Autodesk Inventor part; units mm, degrees
ref_plane "YZ Plane" through (0, 0, 0) normal (1, 0, 0) x (0, 1, 0)
ref_plane "XZ Plane" through (0, 0, 0) normal (0, 1, 0) x (-1, 0, 0)
ref_plane "XY Plane" through (0, 0, 0) normal (0, 0, 1) x (1, 0, 0)
sketch "Skizze1" plane through (0, 0, 0) normal (0, 1, 0) x (-1, 0, 0)
  line L0 (0, 0) -> (15, 0)
  line L1 (15, 0) -> (15, -25)
  line L2 (15, -25) -> (0, -25)
  line L3 (0, -25) -> (0, 0)
  dimension "d0" = 25
  dimension "d1" = 15
extrude "Extrusion1" add sketch "Skizze1" along normal blind 6
sketch "Skizze3" plane through (0, 0, -25) normal (0, 0, -1) x (-1, 0, 0)
  point P0 (0, 0)
sketch "Skizze6" plane through (0, 6, 0) normal (0, 1, 0) x (1, 0, 0)
  circle A0 centre (-11, 5) radius 1.7
  line L0 (-15, 25) -> (-15, 0)
  line L1 (-15, 0) -> (0, 0)
  circle A1 centre (-11, 20) radius 1.7
  line L2 (0, 25) -> (-15, 25)
  point P0 (0, 30)
  dimension "d11" = 3.4
  dimension "d12" = 4
  dimension "d13" = 5
  dimension "d14" = 3.4
  dimension "d15" = 4
  dimension "d16" = 5
extrude "Extrusion4" cut sketch "Skizze6" against normal blind 30
sketch "Skizze7" plane through (0, 0, 0) normal (0, -1, 0) x (1, 0, 0)
  line L0 (0, -25) -> (-15, -25)
  line L1 (0, -25) -> (-7, -25)
  line L2 (-7, -25) -> (-7, -16)
  line L3 (-7, -16) -> (0, -16)
  line L4 (0, -16) -> (0, -25)
  line L5 (-15, 0) -> (0, 0)
  line L6 (0, 0) -> (-7, 0)
  line L7 (-7, 0) -> (-7, -9)
  line L8 (-7, -9) -> (0, -9)
  line L9 (0, -9) -> (0, 0)
  dimension "d19" = 7
  dimension "d20" = 9
  dimension "d21" = 7
  dimension "d22" = 9
extrude "Extrusion5" cut sketch "Skizze7" against normal blind 30
sketch "Skizze8" plane through (-7, 0, -9) normal (0, 0, 1) x (1, 0, 0)
  circle A0 centre (4, 3) radius 1.7
  line L0 (7, 0) -> (0, 0)
  line L1 (7, 6) -> (7, 0)
  dimension "d25" = 3.4
  dimension "d26" = 3
  dimension "d27" = 3
extrude "Extrusion6" cut sketch "Skizze8" against normal blind 30
properties part number "kamera ut" material "CFK"
Input: part model. Units: mm. Frame: model coordinates. A direction names the side the tool comes from. Give positions to 0.01 mm unless a question says otherwise; leave off trailing zeros. Order: outer loops, then holes, each group sorted by start corner. A loop starts at its lowest first (then second) coordinate and runs counter-clockwise, first axis right, second up. Notation, with made-up numbers: (41.25, 37.25) - (92.25, 37.25) arc R18 ccw to (92.25, 62.25) - close; hole circle Ø6 at (57, 7.25). An arc over 180 degrees is marked (long way). Use a Markdown table: item, result.
(1) Pin query (flat end, axial travel): pin 1 (2 mm diameter, centred on x = -11, z = -20, fed in from +Y); pin 2 (1.8 mm diameter, centred on x = -4.5, y = 3.5, fed in from +Z); pin 3 (3 mm diameter, centred on x = -2.5, y = 4.5, fed in from -Z); pin 4 (1.8 mm diameter, centred on y = 4.5, z = -2.5, fed in from +X). Return the tip coordinate at first contact, or that it passes through.
Computed values:
| item | result |
|---|---|
| pin 1 | passes through |
| pin 2 | stops at z = -9 |
| pin 3 | stops at z = -16 |
| pin 4 | stops at x = -7 |
(2) Access query for faces 5 (the flat face through (-5, 3, -16)), 6 (the cylindrical face through (-9.38, 3.04, -20.51)), 7 (the flat face through (-5, 3, -9)). Directions: +Z, -Z, +X, -X, +Y, -Y. A direction counts if a zero-diameter tool reaches every point of the face in a straight line with its end or side. Return the directions, or none.
Computed values:
| item | result |
|---|---|
| face 5 | -Z, +X, +Y, -Y |
| face 6 | +Y, -Y |
| face 7 | +Z, +X, +Y, -Y |
(3) Section query A-A (y = 3). Output: boundary loops of the cut face in (x, z).
Computed values:
| item | result |
|---|---|
| outline | (-15, -25) - (-7, -25) - (-7, -16) - (-4.7, -16) - (-4.7, -9) - (-7, -9) - (-7, 0) - (-15, 0) - close; (-1.3, -16) - (0, -16) - (0, -9) - (-1.3, -9) - close; hole circle Ø3.4 at (-11, -20); hole circle Ø3.4 at (-11, -5) |
(4) Section query D-D (x = -11). Output: boundary loops of the cut face in (y, z).
Computed values:
| item | result |
|---|---|
| outline | (0, -25) - (6, -25) - (6, -21.7) - (0, -21.7) - close; (0, -18.3) - (6, -18.3) - (6, -6.7) - (0, -6.7) - close; (0, -3.3) - (6, -3.3) - (6, 0) - (0, 0) - close |
(5) Section query B-B (x = -3). Output: boundary loops of the cut face in (y, z), then the cut area to 3 significant figures.
Computed values:
| item | result |
|---|---|
| outline | (0, -16) - (1.3, -16) - (1.3, -9) - (0, -9) - close; (4.7, -16) - (6, -16) - (6, -9) - (4.7, -9) - close |
| area | 18.2 mm2 |
(6) Draft query along X for faces 1 (the flat face through (-7, 3, -4)), 2 (the cylindrical face through (-10.2, 3, -3.5)), 3 (the flat face through (-9, 6, -12)), 4 (the cylindrical face through (-1.38, 3.51, -12.45)). Return one class per face: released by +X, released by -X, zero draft, split by the parting line, or undercut.
Computed values:
| item | result |
|---|---|
| face 1 | released by +X |
| face 2 | undercut |
| face 3 | zero draft |
| face 4 | undercut |
(7) Line query: line 1 (Z direction, x = -11, y = 4.25); line 2 (Y direction, x = -3, z = -12); line 3 (X direction, y = 3.75, z = -5). Output: solid intervals per line, ascending. Write a range as from..to.
Computed values:
| item | result |
|---|---|
| line 1 | z = -25..-21.7, -18.3..-6.7, -3.3..0 |
| line 2 | y = 0..1.3, 4.7..6 |
| line 3 | x = -15..-12.7, -9.3..-7 |
(8) Section query C-C (z = -20). Output: boundary loops of the cut face in (x, y).
Computed values:
| item | result |
|---|---|
| outline | (-15, 0) - (-12.7, 0) - (-12.7, 6) - (-15, 6) - close; (-9.3, 0) - (-7, 0) - (-7, 6) - (-9.3, 6) - close |
